```python
from build123d import *

# Parameters (mm, degrees)
SKETCH1_R           = 3.05
BOSS_EXTRUDE1_DEPTH = 10
BOSS_EXTRUDE2_DEPTH = 75.9
SKETCH3_R           = 1.4
CUT_EXTRUDE1_DEPTH  = 6
CHAMFER1_SIZE       = 1.55
CHAMFER2_SIZE       = 2
CHAMFER3_SIZE       = 3.1
CHAMFER4_SIZE       = 3


with BuildPart() as part:
    # Sketch1 → Boss-Extrude1 (new body)
    with BuildSketch(Plane(origin=(0, 0, 0), x_dir=(1, 0, 0), z_dir=(0, 1, 0))):
        Polygon((0, 0), (195, 0), (195, 95), (195, 100.5), (0, 100.5), (0, 95), align=None)
        with Locations(Location((10, 85, 0), (0, 0, 270))):
            Circle(SKETCH1_R, mode=Mode.SUBTRACT)
        with Locations(Location((185, 85, 0), (0, 0, 90))):
            Circle(SKETCH1_R, mode=Mode.SUBTRACT)
        with Locations(Location((185, 10, 0), (0, 0, 270))):
            Circle(SKETCH1_R, mode=Mode.SUBTRACT)
        with Locations(Location((10, 10, 0), (0, 0, 90))):
            Circle(SKETCH1_R, mode=Mode.SUBTRACT)
    extrude(amount=BOSS_EXTRUDE1_DEPTH)

    # Sketch2 → Boss-Extrude2 (add)
    with BuildSketch(Plane(origin=(0, 10, 0), x_dir=(1, 0, 0), z_dir=(0, 1, 0))):
        with BuildLine():
            Line((42.2, 60.5), (89.6, 60.5))
            Line((89.6, 60.5), (89.6, 47.1))
            Line((89.6, 47.1), (156.5, 47.1))
            Line((156.5, 47.1), (156.5, 41.1))
            Line((156.5, 41.1), (164.5, 41.1))
            Line((164.5, 41.1), (164.5, 11.1))
            Line((164.5, 11.1), (156.5, 11.1))
            Line((156.5, 11.1), (156.5, 5.1))
            Line((156.5, 5.1), (40.2, 5.1))
            Line((40.2, 5.1), (40.2, 11.1))
            Line((40.2, 11.1), (32.2, 11.1))
            Line((32.2, 11.1), (32.2, 41.1))
            Line((32.2, 41.1), (40.2, 41.1))
            Line((40.2, 41.1), (40.2, 58.5))
            ThreePointArc((40.2, 58.5), (40.785786438, 59.914213562), (42.2, 60.5))
        make_face()
    extrude(amount=BOSS_EXTRUDE2_DEPTH)

    # Sketch3 → Cut-Extrude1 (cut)
    with BuildSketch(Plane(origin=(0, 85.9, 0), x_dir=(1, 0, 0), z_dir=(0, 1, 0))):
        with Locations(Location((36.2, 33.6, 0), (0, 0, 270))):
            Circle(SKETCH3_R)
        with Locations(Location((36.2, 18.6, 0), (0, 0, 90))):
            Circle(SKETCH3_R)
        with Locations(Location((160.5, 18.6, 0), (0, 0, 270))):
            Circle(SKETCH3_R)
        with Locations(Location((160.5, 33.6, 0), (0, 0, 90))):
            Circle(SKETCH3_R)
    extrude(amount=-CUT_EXTRUDE1_DEPTH, mode=Mode.SUBTRACT)

    # Chamfer1
    chamfer1_edges = [part.edges().sort_by_distance(p)[0] for p in [
        (40.2, 47.95, -41.1),
        (32.2, 47.95, -41.1),
        (32.2, 47.95, -11.1),
        (40.2, 47.95, -11.1),
        (156.5, 47.95, -11.1),
        (164.5, 47.95, -11.1),
        (164.5, 47.95, -41.1),
        (156.5, 47.95, -41.1),
    ]]
    chamfer(chamfer1_edges, length=CHAMFER1_SIZE)

    # Chamfer2
    chamfer2_edges = [part.edges().sort_by_distance(p)[0] for p in [
        (40.2, 47.95, -5.1),
        (156.5, 47.95, -5.1),
        (156.5, 47.95, -47.1),
    ]]
    chamfer(chamfer2_edges, length=CHAMFER2_SIZE)

    # Chamfer3
    chamfer3_edges = [part.edges().sort_by_distance(p)[0] for p in [
        (10, 10, -88.05),
        (185, 10, -81.95),
        (185, 10, -13.05),
        (10, 10, -6.95),
    ]]
    chamfer(chamfer3_edges, length=CHAMFER3_SIZE)

    # Chamfer4
    chamfer4_edges = [part.edges().sort_by_distance(p)[0] for p in [
        (0, 5, -100.5),
        (195, 5, -100.5),
        (195, 5, 0),
        (0, 5, 0),
        (195, 10, -50.25),
        (97.5, 10, -100.5),
        (0, 10, -50.25),
        (97.5, 10, 0),
    ]]
    chamfer(chamfer4_edges, length=CHAMFER4_SIZE)


solid = part.part
```
Check sheet for the modelled part. Datum: model origin and axes. Units: mm. A direction names the side the tool comes from. Round coordinates to 2 decimals unless told otherwise and drop trailing zeros. Order: outer loops, then holes, each group sorted by start corner. A loop starts at its lowest first (then second) coordinate and runs counter-clockwise, first axis right, second up. Notation, with made-up numbers: M 21,33.5 L 52,33.5 A20 cw 52,45.5 Z; hole C 45,48.5 d6. An arc over 180 degrees is marked long. Answer in a Markdown table with one row per item.
(1) Set-up check for faces 5 (the flat face through (122, 47, -47.1)), 6 (the flat face through (32.2, 47, -26)), 7 (the flat face through (161, 47, -11.1)): record each of +Z, -Z, +X, -X, +Y, -Y from which the full face is reachable in a straight line by a thin tool's end or side.
Findings:
| item | result |
|---|---|
| face 5 | -Z, +X, +Y |
| face 6 | +Z, -Z, -X, +Y |
| face 7 | +Z, +X, +Y |
(2) Section check D-D on x = 127.5. Record the boundary of the cut face in (y, z).
Findings:
| item | result |
|---|---|
| outline | M 0,-100.5 L 7,-100.5 L 10,-97.5 L 10,-47.1 L 85.9,-47.1 L 85.9,-5.1 L 10,-5.1 L 10,-3 L 7,0 L 0,0 Z |
(3) Section check B-B on z = -29. Record the boundary of the cut face in (x, y).
Findings:
| item | result |
|---|---|
| outline | M 0,0 L 195,0 L 195,7 L 192,10 L 164.5,10 L 164.5,85.9 L 32.2,85.9 L 32.2,10 L 3,10 L 0,7 Z |
(4) Material ranges on line 1 along Z through (x, y) = (185, 1); line 2 along X through (y, z) = (83.95, -33.6); line 3 along Z through (x, y) = (105.5, 16), recorded low to high. Write a range as from..to.
Findings:
| item | result |
|---|---|
| line 1 | z = -100.5..-88.05, -81.95..-13.05, -6.95..0 |
| line 2 | x = 32.2..34.8, 37.6..159.1, 161.9..164.5 |
| line 3 | z = -47.1..-5.1 |
(5) Section check A-A on x = 10. Record the boundary of the cut face in (y, z).
Findings:
| item | result |
|---|---|
| outline | M 0,-100.5 L 7,-100.5 L 10,-97.5 L 10,-91.15 L 6.9,-88.05 L 0,-88.05 Z; M 0,-81.95 L 6.9,-81.95 L 10,-78.85 L 10,-16.15 L 6.9,-13.05 L 0,-13.05 Z; M 0,-6.95 L 6.9,-6.95 L 10,-3.85 L 10,-3 L 7,0 L 0,0 Z |
(6) Section check C-C on y = 48.5. Record the boundary of the cut face in (x, z), plus the area to 3 significant figures.
Findings:
| item | result |
|---|---|
| outline | M 32.2,-39.55 L 33.75,-41.1 L 38.65,-41.1 L 40.2,-42.65 L 40.2,-58.5 A2 ccw 42.2,-60.5 L 89.6,-60.5 L 89.6,-47.1 L 154.5,-47.1 L 156.5,-45.1 L 156.5,-42.65 L 158.05,-41.1 L 162.95,-41.1 L 164.5,-39.55 L 164.5,-12.65 L 162.95,-11.1 L 158.05,-11.1 L 156.5,-9.55 L 156.5,-7.1 L 154.5,-5.1 L 42.2,-5.1 L 40.2,-7.1 L 40.2,-9.55 L 38.65,-11.1 L 33.75,-11.1 L 32.2,-12.65 Z |
| area | 6,020 mm^2 |
(7) Draft check along Z on faces 1 (the flat face through (96, 10, -61)), 2 (the flat face through (36, 47, -11.1)), 3 (the cylindrical face through (9.866, 3.402, -6.953)), 4 (the cylindrical face through (184.866, 3.402, -81.953)). Enter one of: +Z half, -Z half, draft (parallel to the pull), parting line (faces both ways), or undercut.
Findings:
| item | result |
|---|---|
| face 1 | draft |
| face 2 | +Z half |
| face 3 | undercut |
| face 4 | undercut |
(8) Gauge pin test, flat ends, axial feed: pin 1 (3 mm diameter, centred on y = 74, z = -61.5, fed in from -X); pin 2 (8 mm diameter, centred on y = 45.5, z = -28.5, fed in from -X); pin 3 (1.5 mm diameter, centred on x = 95.5, z = -73.5, fed in from +Y). Record the tip position at first contact, or that the pin passes through.
Findings:
| item | result |
|---|---|
| pin 1 | stops at x = 40.88 |
| pin 2 | stops at x = 32.2 |
| pin 3 | stops at y = 10 |
